For this review, use the dimensioned drawing (mm, ordinates from the lowest corner) and the shaded views. A direction names the side the tool comes from. Give positions to 0.01 mm unless a question says otherwise; leave off trailing zeros. Order: outer loops, then holes, each group sorted by start corner. A loop starts at its lowest first (then second) coordinate and runs counter-clockwise, first axis right, second up. Notation, with made-up numbers: M 49.5,20 L 84.5,20 A30 cw 84.5,42 Z; hole C -28,39.5 d11. An arc over 180 degrees is marked long. One line per question, with ' | ' between items. Start each with the question number.
1. The part is to be moulded in two halves that separate along X. For the marked faces 4, 5, 6 and 7, say which applies: +X half, -X half, draft (parallel to the pull), parting line (faces both ways), or undercut.
2. Insertion check: P1, Ø10, axis at y = 18, z = 32.5, coming from the -X side; P2, Ø25, axis at y = 21.5, z = 42, coming from the -X side; P3, Ø3, axis at y = 33, z = 41.5, coming from the -X side. Each pin has a flat end and moves straight along its axis. Give the tip position at first contact, or say it passes through.
3. We need section A-A on y = 13. Write out the cut boundary in (x, z), then the cut area to 3 significant figures.
4. We need section D-D on y = 47. Write out the cut boundary in (x, z).
5. We need section C-C on z = 60. Write out the cut boundary in (x, y), then the cut area to 3 significant figures.
6. We need section B-B on z = 19. Write out the cut boundary in (x, y) (1 decimal), then the cut area to 3 significant figures.
7. For the marked faces 1, 2 and 3, list the 3-axis set-ups (+Z, -Z, +X, -X, +Y, -Y) from which the entire face can be reached by the end or side of a thin tool; tool diameter is ignored.
8. Wall thickness on L1, parallel to X at y = 47, z = 22; L2, parallel to Z at x = 6, y = 13; L3, parallel to X at y = 26, z = 14: over which ranges is each line inside the solid? List them lowest first.
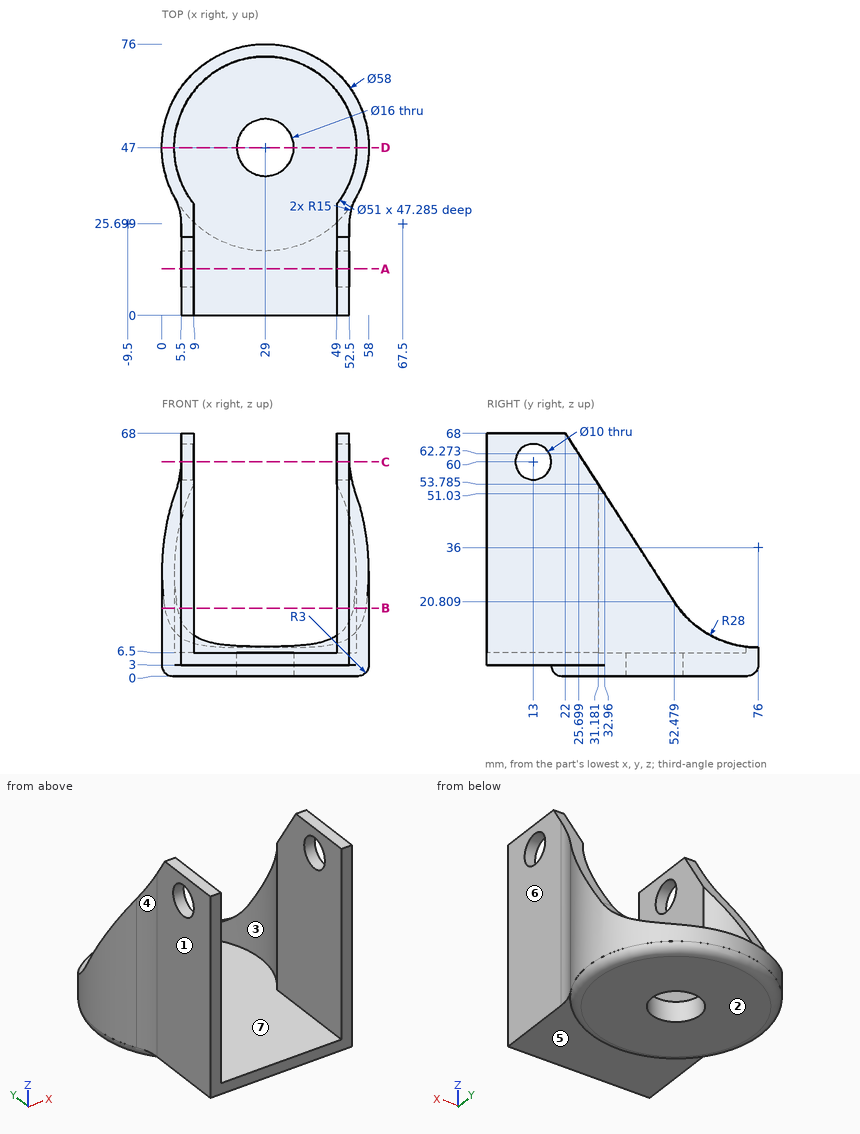
Entries:
1) face 4: -X half | face 5: draft | face 6: +X half | face 7: undercut
2) P1: stops at x = 5.5 | P2: stops at x = 3.08 | P3: stops at x = 2.83
3) outline: M 5.5,3 L 52.5,3 L 52.5,55 L 49,55 L 49,6.5 L 9,6.5 L 9,55 L 5.5,55 Z; M 5.5,65 L 9,65 L 9,68 L 5.5,68 Z; M 49,65 L 52.5,65 L 52.5,68 L 49,68 Z | area: 525 mm^2
4) outline: M 0,3 A3 ccw 3,0 L 21,0 L 21,6.5 L 3.5,6.5 L 3.5,29.29 L 0,29.29 Z; M 37,0 L 55,0 A3 ccw 58,3 L 58,29.29 L 54.5,29.29 L 54.5,6.5 L 37,6.5 Z
5) outline: M 5.43,27.17 A15 cw 5.5,25.7 L 5.5,18 L 9,18 L 9,27.17 Z; M 5.5,0 L 9,0 L 9,8 L 5.5,8 Z; M 49,0 L 52.5,0 L 52.5,8 L 49,8 Z; M 49,18 L 52.5,18 L 52.5,25.7 A15 cw 52.57,27.17 L 49,27.17 Z | area: 120 mm^2
6) outline: M 0.8,53.8 A29 ccw 3.6,33 A15 cw 5.5,25.7 L 5.5,0 L 9,0 L 9,31.2 A25.5 cw 4.4,53.8 Z; M 49,0 L 52.5,0 L 52.5,25.7 A15 cw 54.4,33 A29 ccw 57.2,53.8 L 53.6,53.8 A25.5 cw 49,31.2 Z | area: 388 mm^2
7) face 1: +Z, -Z, -X, -Y | face 2: -Z, +X, -X, +Y, -Y | face 3: +Z
8) L1: x = 0 to 3.5, 54.5 to 58 | L2: z = 3 to 55, 65 to 68 | L3: x = 5.5 to 9, 49 to 52.5
